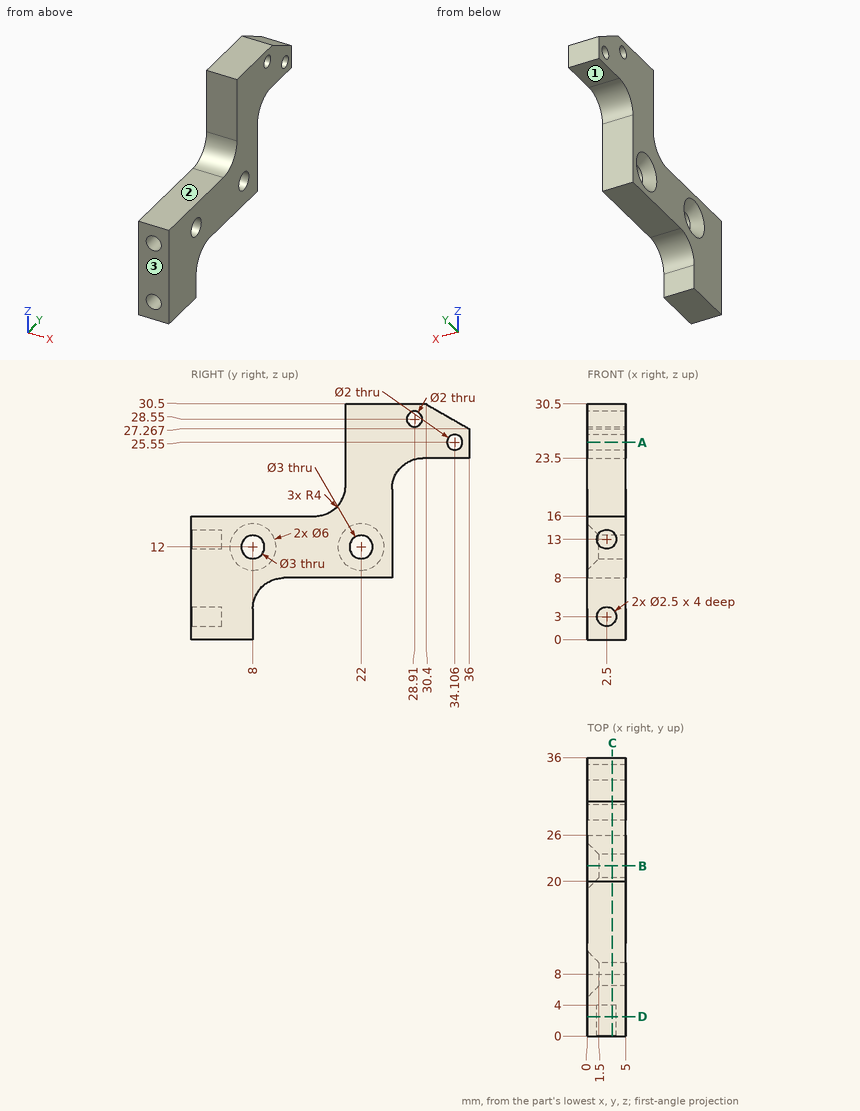
Input: dimensioned drawing with shaded views. Units: mm. Origin: part minimum x, y, z. A direction names the side the tool comes from. Coordinates: 2 decimals unless noted, no trailing zeros. Loops run counter-clockwise (first coordinate to the right, second up) from the corner with the lowest first, then second, coordinate; pieces in that order, holes last. Notation, with made-up numbers: M 52.25,8 L 108.25,8 A16 ccw 108.25,21 Z; hole C 54,43 d5. An arc over 180 degrees is marked long. Use a Markdown table: item, result. Add a question column.
1) Set-up query: the marked faces 1, 2 and 3. Return all of +Z, -Z, +X, -X, +Y, -Y with unobstructed straight access to the full face (end or side cutting, diameter ignored); none if empty.
2) Pin query (flat end, axial travel): P1, Ø2.5, axis at x = 3.5, y = 5, coming from the +Z side; P2, Ø2, axis at x = 2.5, z = 3, coming from the -Y side; P3, Ø1.5, axis at x = 3, z = 15, coming from the +Y side; P4, Ø3, axis at y = 34.11, z = 25.55, coming from the +X side. Return the tip coordinate at first contact, or that it passes through.
3) Section A-A, the plane z = 25.55. Return the cut outline in (x, y).
4) Section C-C, the plane x = 3.25. Return the cut outline in (y, z), plus the area to 3 significant figures.
5) Section D-D, the plane y = 2.5. Return the cut outline in (x, z).
6) Line query: L1, parallel to Y at x = 3.85, z = 12; L2, parallel to Y at x = 3, z = 12; L3, parallel to Z at x = 2.5, y = 2. Output: solid intervals per line, ascending. Write a range as from..to.
7) Section B-B, the plane y = 22. Return the cut outline in (x, z).
Answer below:
| question | item | result |
|---|---|---|
| 1 | face 1 | -Z, +X, -X, +Y |
| 1 | face 2 | +Z, +X, -X, -Y |
| 1 | face 3 | +Z, -Z, +X, -X, -Y |
| 2 | P1 | z = 16 |
| 2 | P2 | y = 4 |
| 2 | P3 | y = 26 |
| 2 | P4 | x = 5 |
| 3 | outline | M 0,20 L 5,20 L 5,33.11 L 0,33.11 Z; M 0,35.11 L 5,35.11 L 5,36 L 0,36 Z |
| 4 | outline | M 0,0 L 8,0 L 8,4 A4 cw 12,8 L 26,8 L 26,19.5 A4 cw 30,23.5 L 36,23.5 L 36,27.27 L 30.4,30.5 L 20,30.5 L 20,20 A4 cw 16,16 L 0,16 L 0,14 L 4,14 L 4,12 L 0,12 L 0,4 L 4,4 L 4,2 L 0,2 Z; hole C 8,12 d3; hole C 22,12 d3; hole C 28.91,28.55 d2; hole C 34.11,25.55 d2 |
| 4 | area | 394 mm2 |
| 5 | outline | M 0,0 L 5,0 L 5,16 L 0,16 Z; hole C 2.5,3 d2.5; hole C 2.5,13 d2.5 |
| 6 | L1 | 0..6.5, 9.5..20.5, 23.5..26 |
| 6 | L2 | 4..6.5, 9.5..20.5, 23.5..26 |
| 6 | L3 | 0..1.75, 4.25..11.75, 14.25..16 |
| 7 | outline | M 0,8 L 5,8 L 5,10.5 L 1.5,10.5 L 0,9 Z; M 0,15 L 1.5,13.5 L 5,13.5 L 5,30.5 L 0,30.5 Z |
